from build123d import *

# Parameters (mm, degrees)
F0_R     = 25
F1_DEPTH = 100
F2_DEPTH = 25
F3_R     = 25
F3_W     = 22.6668892428
F3_H     = 19.8441343382
F4_DEPTH = 25


with BuildPart() as f1:
    # F0 (on Front) → F1 (new body)
    with BuildSketch(Plane.XZ):
        Circle(F0_R)
    extrude(amount=F1_DEPTH)

    # F2 (add): a face of the model
    f2_faces = [f1.faces().sort_by_distance(p)[0] for p in [
        (0, -100, 0),
    ]]
    extrude(f2_faces, amount=F2_DEPTH)

    # F3 (on face) → F4 (join)
    with BuildSketch(Plane.XZ.offset(125)):
        Circle(F3_R)
        with Locations((2.1329852752, -3.9242249914)):
            Rectangle(F3_W, F3_H, mode=Mode.SUBTRACT)
    extrude(amount=F4_DEPTH)


solid = f1.part
Model file for the job. Use its own axes, mm. A direction names the side the tool comes from. Coordinates: 2 decimals unless noted, no trailing zeros. Loops run counter-clockwise (first coordinate to the right, second up) from the corner with the lowest first, then second, coordinate; pieces in that order, holes last. Notation, with made-up numbers: (-26.75, 65.25) -> (24.25, 65.25) arc R12 cw to (24.25, 79.25) -> close; hole circle Ø10 at (82.5, -10). An arc over 180 degrees is marked (long way). Use one line per item in the form item = value. Start each with the question number.
(1) Flat gauge pins, fed straight in: pin 1 (18 mm diameter, centred on x = -0.5, y = -132.5, fed in from +Z); pin 2 (1.5 mm diameter, centred on x = -18, y = -83, fed in from -Z); pin 3 (1 mm diameter, centred on y = -53, z = -16.5, fed in from -X). Where does each tip first touch, or does it go through?
(2) Cut at A-A on x = 0. Give the cut face in (y, z).
(3) Cut at C-C on y = -72. Give the cut face in (x, z), and give its area (3 significant figures).
(4) Cut at D-D on z = 20. Give the cut face in (x, y), and give its area (3 significant figures).
(5) Tool access for faces 4 (the flat face through (0, 0, 0)), 5 (the flat face through (2, -137, -13.846)): list every direction of +Z, -Z, +X, -X, +Y, -Y with a clear straight run to the whole face (end or side of a thin tool).
(6) Cut at B-B on z = 0. Give the cut face in (x, y), and give its area (3 significant figures).
(7) Probe probe 1 along Y at (x, z) = (9, -3.5); probe 2 along Z at (x, y) = (-15.5, -84.5); probe 3 along X at (y, z) = (-19.5, 9). List the from-to ranges inside material, lowest first. Write a range as from..to.
(8) Pull direction X, two halves, no side cores. Call faces 1 (the cylindrical face through (23.846, -73.95, 7.509)), 2 (the flat face through (-11, -150, 0)), 3 (the flat face through (13.466, -137, -4)): pulls with the +X half, pulls with the -X half, needs draft (parallel to the pull), parting line crosses it, or undercut.
Values:
q1.pin_1 = 25
q1.pin_2 = -18.1
q1.pin_3 = -19.21
q2.outline = (-150, -25) -> (0, -25) -> (0, 25) -> (-150, 25) -> (-150, 6) -> (-125, 6) -> (-125, -13.85) -> (-150, -13.85) -> close
q3.outline = circle Ø50 at (0, 0)
q3.area = 1,960 mm2
q4.outline = (-15, -150) -> (15, -150) -> (15, 0) -> (-15, 0) -> close
q4.area = 4,500 mm2
q5.face_4 = +Z, -Z, +X, -X, +Y
q5.face_5 = -Y
q6.outline = (-25, -150) -> (-9.2, -150) -> (-9.2, -125) -> (13.47, -125) -> (13.47, -150) -> (25, -150) -> (25, 0) -> (-25, 0) -> close
q6.area = 6,930 mm2
q7.probe_1 = -125..0
q7.probe_2 = -19.62..19.62
q7.probe_3 = -23.32..23.32
q8.face_1 = parting line crosses it
q8.face_2 = needs draft
q8.face_3 = undercut
